The figure shows three views and two pictorial views of one solid part (mm, origin at its lowest corner). Answer the questions. Round coordinates to 2 decimals unless told otherwise and drop trailing zeros. Write each loop counter-clockwise with the first axis right and the second up, starting at its lowest first coordinate (ties: lowest second). Pieces come first, ordered by that corner, then holes.
Item 1: Each of these flat-tipped pins is pushed along its axis until it touches: pin 1 (4 mm diameter, centred on y = 13.5, z = 53, fed in from +X); pin 2 (10 mm diameter, centred on x = 385.5, y = 15, fed in from -Z). Where does it stop, or does it pass through?
Item 2: Find section D-D on z = 60.5. Give the vertices of the cut face in (x, y), then the cut area to 3 significant figures.
Item 3: Find section C-C on y = 10.5. Give the vertices of the cut face in (x, z).
Item 4: Find section A-A on x = 162.5. Give the vertices of the cut face in (y, z), then the cut area to 3 significant figures.
Item 5: Find the intervals of material crossed by probe 1 along Z at (x, y) = (330.5, 16.25); probe 2 along X at (y, z) = (8.5, 153.5); probe 3 along Z at (x, y) = (373, 8.75), in increasing order.
Item 6: Find section B-B on z = 250.5. Give the vertices of the cut face in (x, y).
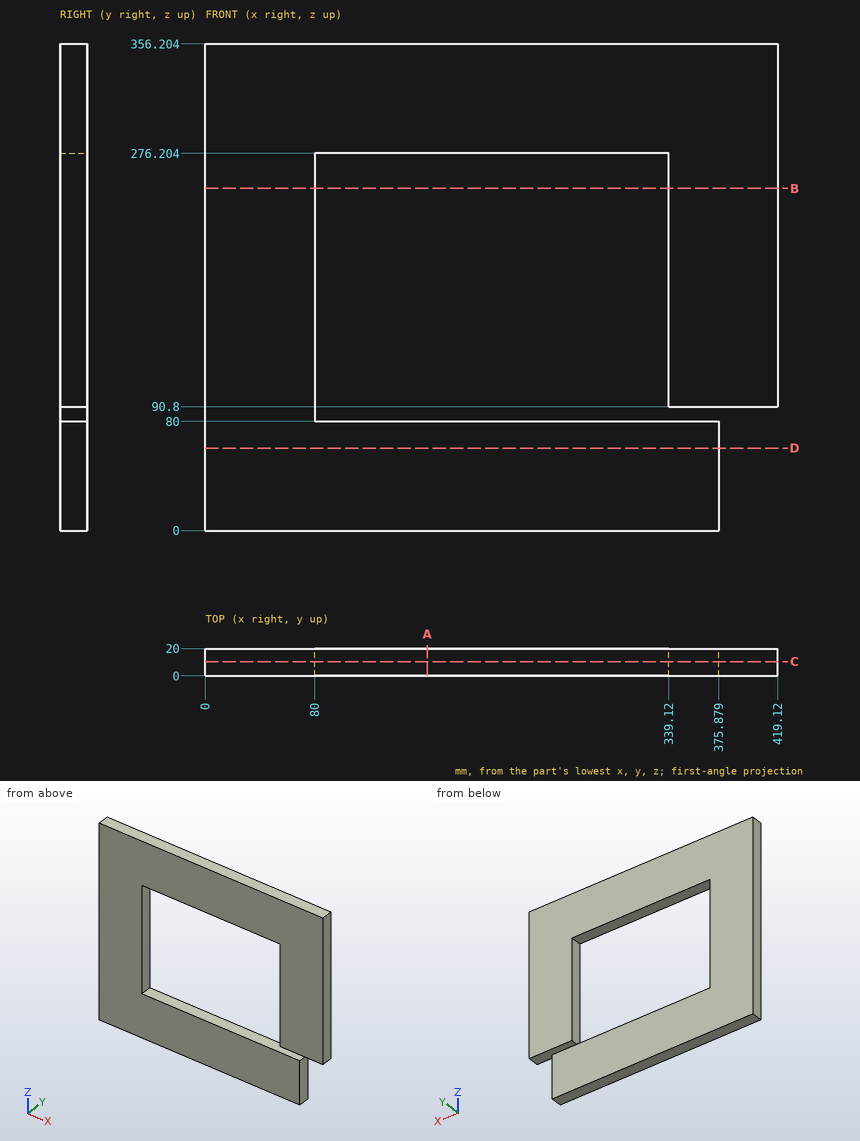
Check values:
1. pin 1: stops at x = 375.88
1. pin 2: stops at z = 90.8
2. outline: (0, 0) - (375.88, 0) - (375.88, 20) - (0, 20) - close
2. area: 7,520 mm2
3. outline: (0, 0) - (375.88, 0) - (375.88, 80) - (80, 80) - (80, 276.2) - (339.12, 276.2) - (339.12, 90.8) - (419.12, 90.8) - (419.12, 356.2) - (0, 356.2) - close
4. outline: (0, 0) - (20, 0) - (20, 80) - (0, 80) - close; (0, 276.2) - (20, 276.2) - (20, 356.2) - (0, 356.2) - close
4. area: 3,200 mm2
5. probe 1: z = 0 to 80, 276.2 to 356.2
5. probe 2: x = 0 to 80, 339.12 to 419.12
5. probe 3: z = 0 to 80, 90.8 to 356.2
6. outline: (0, 0) - (80, 0) - (80, 20) - (0, 20) - close; (339.12, 0) - (419.12, 0) - (419.12, 20) - (339.12, 20) - close
